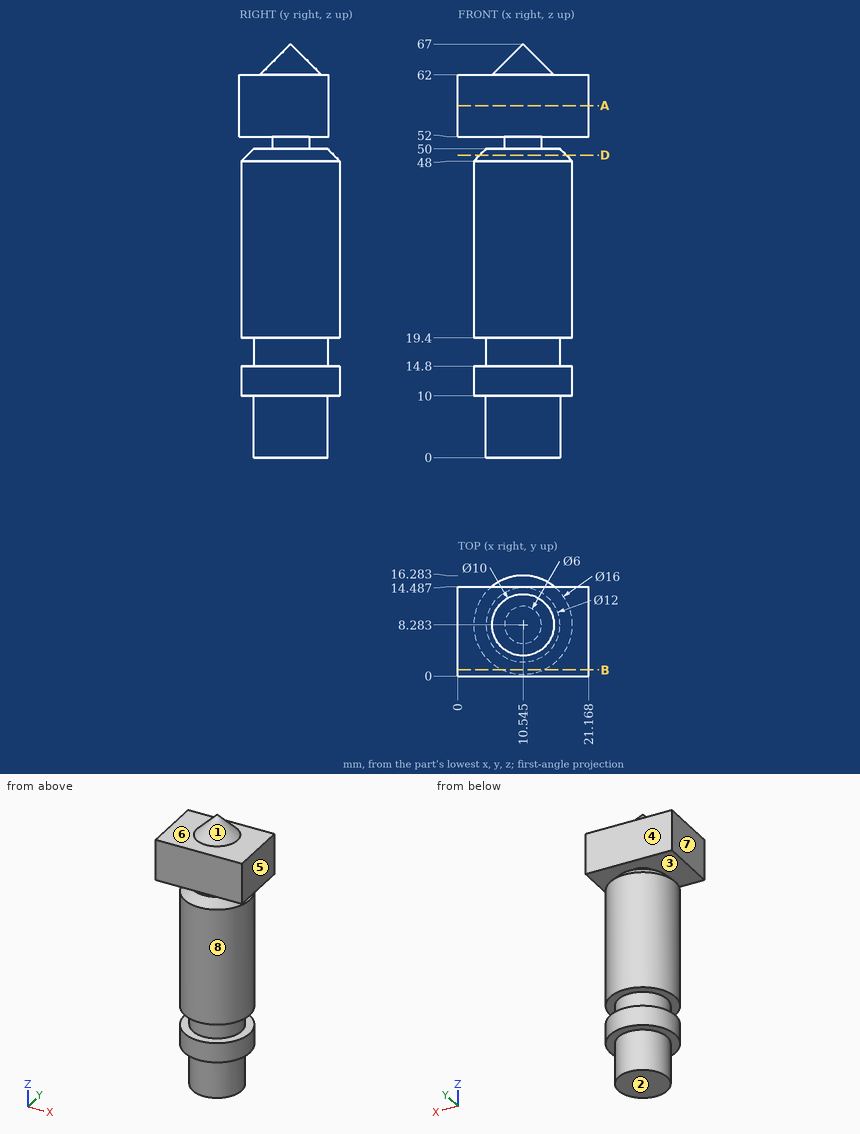
Check sheet for the drawn part. Datum: minimum x, y, z corner. Units: mm. A direction names the side the tool comes from. Round coordinates to 2 decimals unless told otherwise and drop trailing zeros. Loops run counter-clockwise (first coordinate to the right, second up) from the corner with the lowest first, then second, coordinate; pieces in that order, holes last.
Item 1: Cross-section at B-B on y = 1. Count the separate pieces of the cut face and the enclosed holes in it, then the cut area to 3 significant figures.
Item 2: Mould release check, pull along Z, two halves, no side actions. Record for the marked faces 1, 2 and 3: pulls with the +Z half, pulls with the -Z half, needs draft (parallel to the pull), parting line crosses it, or undercut.
Item 3: Access from +Z, -Z, +X, -X, +Y, -Y to the whole of each face (thin tool, end or side, straight path). Record for the marked faces 4, 5, 6, 7 and 8.
Item 4: Cross-section at D-D on z = 49. Record the boundary of the cut face in (x, y) (1 decimal), then the cut area to 3 significant figures.
Item 5: Gauge pin test, flat ends, axial feed: pin 1 (4 mm diameter, centred on x = 14, y = 9, fed in from +Z); pin 2 (3.5 mm diameter, centred on x = 13, y = 11, fed in from +Z); pin 3 (1 mm diameter, centred on x = 5.5, z = 58, fed in from +Y). Record the tip position at first contact, or that the pin passes through.
Item 6: Thickness scan on line 1 (Z direction, x = 11.25, y = 2.75); line 2 (Z direction, x = 2.75, y = 8.5) (1 decimal); line 3 (Y direction, x = 15.5, z = 59). Record the ranges inside material, lowest first.
Item 7: Cross-section at A-A on z = 57. Record the boundary of the cut face in (x, y).
Answer sheet:
1. separate pieces: 3
1. enclosed holes: 0
1. area: 436 mm2
2. face 1: pulls with the +Z half
2. face 2: pulls with the -Z half
2. face 3: undercut
3. face 4: +Z, +X, -X, +Y
3. face 5: +Z, -Z, +X, +Y, -Y
3. face 6: +Z
3. face 7: +Z, -Z, -X, +Y, -Y
3. face 8: -Z
4. outline: circle Ø14 at (10.5, 8.3)
4. area: 154 mm2
5. pin 1: stops at z = 65.47
5. pin 2: stops at z = 65.09
5. pin 3: stops at y = 14.49
6. line 1: z = 0 to 50, 52 to 62
6. line 2: z = 10 to 14.8, 19.4 to 48.2, 52 to 62
6. line 3: y = 0 to 14.49
7. outline: (0, 0) - (21.17, 0) - (21.17, 14.49) - (0, 14.49) - close
